Autodesk Inventor part; units mm, degrees
ref_plane "YZ Plane" through (0, 0, 0) normal (1, 0, 0) x (0, 1, 0)
ref_plane "XZ Plane" through (0, 0, 0) normal (0, 1, 0) x (-1, 0, 0)
ref_plane "XY Plane" through (0, 0, 0) normal (0, 0, 1) x (1, 0, 0)
sketch "Sketch1" plane through (0, 0, 0) normal (0, 0, 1) x (1, 0, 0)
  circle A0 centre (-74.1769, -5.2291) radius 2.1844
  circle A1 centre (-112.2444, -5.4371) radius 2.1844
  circle A2 centre (-94.297, -37.5832) radius 2.1844
  circle A3 centre (-54.0602, 27.1276) radius 2.1844
  arc A4 (-100.6091, -36.8907) -> (-114.967, -11.1738) centre (-125.8576, -34.1206) ccw
  arc A5 (-112.8432, 0.8846) -> (-59.1316, 30.942) centre (-120.0293, 76.745) ccw
  arc A6 (-112.8432, 0.8846) -> (-114.967, -11.1738) centre (-112.2444, -5.4371) ccw
  line L0 (-88.9043, -40.936) -> (-48.6711, 23.7771)
  arc A7 (-48.6711, 23.7771) -> (-59.1316, 30.942) centre (-54.0602, 27.1276) ccw
  arc A8 (-100.6091, -36.8907) -> (-88.9043, -40.936) centre (-94.297, -37.5832) ccw
  dimension "d6" = 25.4
  dimension "d8" = 76.2
extrude "Extrusion3" add sketch "Sketch1" along normal blind 1.5875
properties part number "Side Poly"
Check sheet for the modelled part. Datum: model origin and axes. Units: mm. Coordinates: 2 decimals unless noted, no trailing zeros. Loops run counter-clockwise (first coordinate to the right, second up) from the corner with the lowest first, then second, coordinate; pieces in that order, holes last. Notation, with made-up numbers: (-31, 73) -> (24, 73) arc R23 ccw to (24, 105) -> close; hole circle Ø4 at (60, 6.25). An arc over 180 degrees is marked (long way). Write item = value, one per line. Start each with the question number.
1. Section check A-A on x = -53. Record the cut outline in (y, z), then the cut area to 3 significant figures.
2. Draft check along X on faces 1 (the cylindrical face through (-93.289, -35.645, 0.783)), 2 (the flat face through (-69.07, -9.03, 0.78)), 3 (the cylindrical face through (-103.788, -21.547, 0.783)), 4 (the flat face through (-84, -5, 1.588)). Enter one of: released by +X, released by -X, zero draft, split by the parting line, or undercut.
3. Material ranges on line 1 (X direction, y = -6, z = 1.1); line 2 (Y direction, x = -96, z = 0.95); line 3 (X direction, y = -38, z = 1.05), recorded low to high.
4. Section check B-B on z = 1.1. Record the cut outline in (x, y).
5. Section check D-D on x = -94. Record the cut outline in (y, z), then the cut area to 3 significant figures.
6. Depth check by flat-ended pin: P1, Ø7, axis at x = -74.18, y = -5.23, coming from the -Z side. Enter the tip coordinate at first touch or a pass-through.
7. Section check C-C on y = -28. Record the cut outline in (x, z), then the cut area to 3 significant figures.
Responses:
q1.outline = (16.81, 0) -> (25.22, 0) -> (25.22, 1.59) -> (16.81, 1.59) -> close; (29.04, 0) -> (33.38, 0) -> (33.38, 1.59) -> (29.04, 1.59) -> close
q1.area = 20.2 mm2
q2.face_1 = undercut
q2.face_2 = released by +X
q2.face_3 = released by -X
q2.face_4 = zero draft
q3.line_1 = -118.57 to -114.36, -110.13 to -76.22, -72.13 to -67.18
q3.line_2 = -43.7 to -38.95, -36.22 to 4.43
q3.line_3 = -100.63 to -96.44, -92.15 to -87.08
q4.outline = (-114.97, -11.17) arc R25.4 cw to (-100.61, -36.89) arc R6.35 ccw to (-88.9, -40.94) -> (-48.67, 23.78) arc R6.35 ccw to (-59.13, 30.94) arc R76.2 cw to (-112.84, 0.88) arc R6.35 ccw to start; hole circle Ø4.37 at (-112.24, -5.44); hole circle Ø4.37 at (-94.3, -37.58); hole circle Ø4.37 at (-74.18, -5.23); hole circle Ø4.37 at (-54.06, 27.13)
q5.outline = (-43.93, 0) -> (-39.75, 0) -> (-39.75, 1.59) -> (-43.93, 1.59) -> close; (-35.42, 0) -> (5.13, 0) -> (5.13, 1.59) -> (-35.42, 1.59) -> close
q5.area = 71.0 mm2
q6.P1 = 0
q7.outline = (-101.21, 0) -> (-80.86, 0) -> (-80.86, 1.59) -> (-101.21, 1.59) -> close
q7.area = 32.3 mm2
